```python
from build123d import *

# Parameters (mm, degrees)
SKETCH_1_W          = 140
SKETCH_1_H          = 103
EXTRUDE_1_DEPTH     = 0.5
CUT_EXTRUDE_1_DEPTH = 1.5
CUT_EXTRUDE_2_DEPTH = 1.5
SKETCH_4_W          = 33.363809018
SKETCH_4_H          = 55
CUT_EXTRUDE_3_DEPTH = 1
FILLET_1_R          = 2
SKETCH_6_R          = 1.525
CUT_EXTRUDE_5_DEPTH = 10
SKETCH_7_R          = 1.525
CUT_EXTRUDE_6_DEPTH = 10
SKETCH_8_R          = 1.525
SKETCH_8_W          = 39.445445888
SKETCH_8_H          = 5
CUT_EXTRUDE_7_DEPTH = 10
FILLET_2_R          = 1


with BuildPart() as part:
    # 草图1 → 凸台-拉伸1 (new, symmetric)
    with BuildSketch(Plane.XY):
        Rectangle(SKETCH_1_W, SKETCH_1_H)
    extrude(amount=EXTRUDE_1_DEPTH, both=True)

    # 草图2 → 切除-拉伸1 (cut, symmetric)
    with BuildSketch(Plane.XY.offset(0.5)):
        with BuildLine():
            Line((-71.445445888, -29.5), (-71.445445888, -77.5))
            ThreePointArc((-71.445445888, -77.5), (-69.980979794, -81.035533906), (-66.445445888, -82.5))
            Line((-66.445445888, -82.5), (-42.445445888, -82.5))
            ThreePointArc((-42.445445888, -82.5), (-38.909911982, -81.035533906), (-37.445445888, -77.5))
            Line((-37.445445888, -77.5), (-37.445445888, -29.5))
            ThreePointArc((-37.445445888, -29.5), (-34.619011221, -12.115704179), (-26.430867135, 3.477780697))
            ThreePointArc((-26.430867135, 3.477780697), (-26.030895398, 11.934357254), (-33.750115979, 15.411036429))
            ThreePointArc((-33.750115979, 15.411036429), (-60.772664783, -0.183029274), (-71.445445888, -29.5))
        make_face()
        with BuildLine():
            Line((6, -82.5), (34, -82.5))
            ThreePointArc((34, -82.5), (36.828427125, -81.328427125), (38, -78.5))
            Line((38, -78.5), (38, -0.5))
            ThreePointArc((38, -0.5), (36.828427125, 2.328427125), (34, 3.5))
            Line((34, 3.5), (6, 3.5))
            ThreePointArc((6, 3.5), (3.171572875, 2.328427125), (2, -0.5))
            Line((2, -0.5), (2, -78.5))
            ThreePointArc((2, -78.5), (3.171572875, -81.328427125), (6, -82.5))
        make_face()
    extrude(amount=CUT_EXTRUDE_1_DEPTH, both=True, mode=Mode.SUBTRACT)

    # 草图3 → 切除-拉伸2 (cut, symmetric)
    with BuildSketch(Plane.XY.offset(0.5)):
        Polygon((67.363809018, -51.5), (39.765042197, 51.5), (70, 51.5), (70, -51.5), align=None)
    extrude(amount=CUT_EXTRUDE_2_DEPTH, both=True, mode=Mode.SUBTRACT)

    # 草图4 → 切除-拉伸3 (cut, symmetric)
    with BuildSketch(Plane.XY.offset(0.5)):
        with Locations((50.681904509, -24)):
            Rectangle(SKETCH_4_W, SKETCH_4_H)
    extrude(amount=CUT_EXTRUDE_3_DEPTH, both=True, mode=Mode.SUBTRACT)

    # 圆角1
    fillet_1_edges = [part.edges().sort_by_distance(p)[0] for p in [
        (-70, -18.109646868, 0),
    ]]
    fillet(fillet_1_edges, radius=FILLET_1_R)

    # 草图6 → 切除-拉伸5 (cut)
    with BuildSketch(Plane.XY.offset(0.5)):
        with Locations((-26, 47.5)):
            Circle(SKETCH_6_R)
        with Locations((-6, 47.5)):
            Circle(SKETCH_6_R)
    extrude(amount=-CUT_EXTRUDE_5_DEPTH, mode=Mode.SUBTRACT)

    # 草图7 → 切除-拉伸6 (cut)
    with BuildSketch(Plane(origin=(0, 0, -0.5), x_dir=(-1, 0, 0), z_dir=(0, 0, -1))):
        with Locations((67, 6.5)):
            Circle(SKETCH_7_R)
        with Locations((67, 26.5)):
            Circle(SKETCH_7_R)
    extrude(amount=-CUT_EXTRUDE_6_DEPTH, mode=Mode.SUBTRACT)

    # 草图8 → 切除-拉伸7 (cut)
    with BuildSketch(Plane.XY.offset(0.5)):
        with Locations((-23.45, -43.5)):
            Circle(SKETCH_8_R)
        with Locations((-3.45, -43.5)):
            Circle(SKETCH_8_R)
        with Locations((-17.722722944, -49)):
            Rectangle(SKETCH_8_W, SKETCH_8_H)
    extrude(amount=-CUT_EXTRUDE_7_DEPTH, mode=Mode.SUBTRACT)

    # 圆角2
    fillet_2_edges = [part.edges().sort_by_distance(p)[0] for p in [
        (52.626603434, 3.5, 0),
        (-37.445445888, -46.5, 0),
        (2, -46.5, 0),
        (-70, 51.5, 0),
        (39.765042197, 51.5, 0),
    ]]
    fillet(fillet_2_edges, radius=FILLET_2_R)


solid = part.part
```
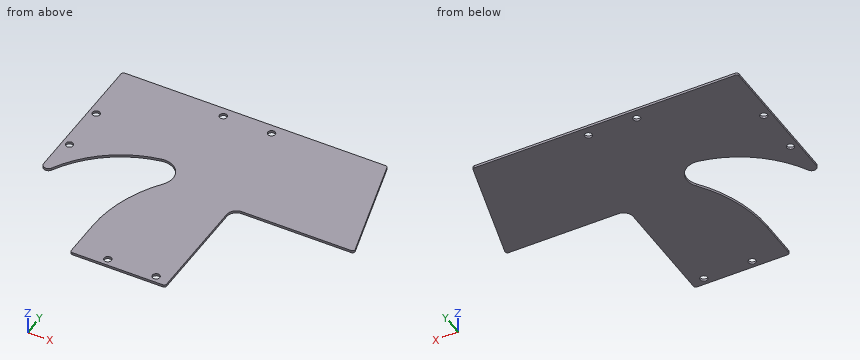
Work out the finished part from the listing and answer in its coordinate system (mm). Give positions to 0.01 mm unless a question says otherwise; leave off trailing zeros. Loops run counter-clockwise (first coordinate to the right, second up) from the corner with the lowest first, then second, coordinate; pieces in that order, holes last. Notation, with made-up numbers: (-29.75, -35) -> (-12.75, -35) arc R16 ccw to (-12.75, -23) -> close; hole circle Ø6 at (-12, -5). An arc over 180 degrees is marked (long way). Use CSV: the item, a comma, the result in double quotes.
1. Straight lines are drawn through the part: line 1 (Y direction, x = -27, z = 0.35); line 2 (Y direction, x = -67, z = -0.2) (3 decimals); line 3 (Y direction, x = -6, z = 0.1) (3 decimals). For each, find the intervals that lie inside material, in ascending order.
Found:
line 1,"-46.5 to 2.71, 13.19 to 46.35, 48.65 to 51.5"
line 2,"-9.124 to 4.975, 8.025 to 24.975, 28.025 to 51.5"
line 3,"-46.5 to 45.975, 49.025 to 51.5"
2. Flat-ended cylindrical pins translate along their axes: pin 1 Ø1.8 at (x, y) = (-6, 47.5) entering from +Z; pin 2 Ø3.5 at (x, y) = (-3.45, -43.5) entering from +Z; pin 3 Ø0.5 at (x, z) = (32, 0) entering from -Y. Find the tip coordinate at first contact, or state that the pin passes through.
Found:
pin 1,"through"
pin 2,"z = 0.5"
pin 3,"y = 3.5"
3. The part is cut by section D-D (y = 47.5). Write down the section's boundary in (x, z) (3 decimals), then the cut area to 3 significant figures.
Found:
outline,"(-70, -0.5) -> (-27.525, -0.5) -> (-27.525, 0.5) -> (-70, 0.5) -> close; (-24.475, -0.5) -> (-7.525, -0.5) -> (-7.525, 0.5) -> (-24.475, 0.5) -> close; (-4.475, -0.5) -> (40.837, -0.5) -> (40.837, 0.5) -> (-4.475, 0.5) -> close"
area,"105 mm^2"
4. The part is cut by section B-B (z = -0.3). Write down the section's boundary in (x, y) (3 decimals), then the cut area to 3 significant figures.
Found:
outline,"(-70, -7.392) arc R2 ccw to (-66.229, -8.321) arc R45.602 cw to (-33.75, 15.411) arc R7.525 cw to (-26.431, 3.478) arc R54.875 ccw to (-37.445, -29.5) -> (-37.445, -45.5) arc R1 ccw to (-36.445, -46.5) -> (1, -46.5) arc R1 ccw to (2, -45.5) -> (2, -0.5) arc R4 cw to (6, 3.5) -> (51.323, 3.5) arc R1 ccw to (52.289, 4.759) -> (39.964, 50.759) arc R1 ccw to (38.998, 51.5) -> (-69, 51.5) arc R1 ccw to (-70, 50.5) -> close; hole circle Ø3.05 at (-67, 6.5); hole circle Ø3.05 at (-67, 26.5); hole circle Ø3.05 at (-26, 47.5); hole circle Ø3.05 at (-23.45, -43.5); hole circle Ø3.05 at (-6, 47.5); hole circle Ø3.05 at (-3.45, -43.5)"
area,"7,220 mm^2"
5. The part is cut by section A-A (y = -43.5). Write down the section's boundary in (x, z) (3 decimals).
Found:
outline,"(-37.445, -0.5) -> (-24.975, -0.5) -> (-24.975, 0.5) -> (-37.445, 0.5) -> close; (-21.925, -0.5) -> (-4.975, -0.5) -> (-4.975, 0.5) -> (-21.925, 0.5) -> close; (-1.925, -0.5) -> (2, -0.5) -> (2, 0.5) -> (-1.925, 0.5) -> close"
6. The part is cut by section C-C (y = 26.5). Write down the section's boundary in (x, z) (3 decimals), then the cut area to 3 significant figures.
Found:
outline,"(-70, -0.5) -> (-68.525, -0.5) -> (-68.525, 0.5) -> (-70, 0.5) -> close; (-65.475, -0.5) -> (46.464, -0.5) -> (46.464, 0.5) -> (-65.475, 0.5) -> close"
area,"113 mm^2"
